Here's the drawing with two shaded views (mm, measured from the low corner). I have some questions. A direction names the side the tool comes from. Round coordinates to 2 decimals unless told otherwise and drop trailing zeros. Order: outer loops, then holes, each group sorted by start corner. A loop starts at its lowest first (then second) coordinate and runs counter-clockwise, first axis right, second up. Notation, with made-up numbers: M 71,33.25 L 108,33.25 A21 ccw 108,60.25 Z; hole C -39,22 d8. An arc over 180 degrees is marked long. One line per question, with ' | ' between items.
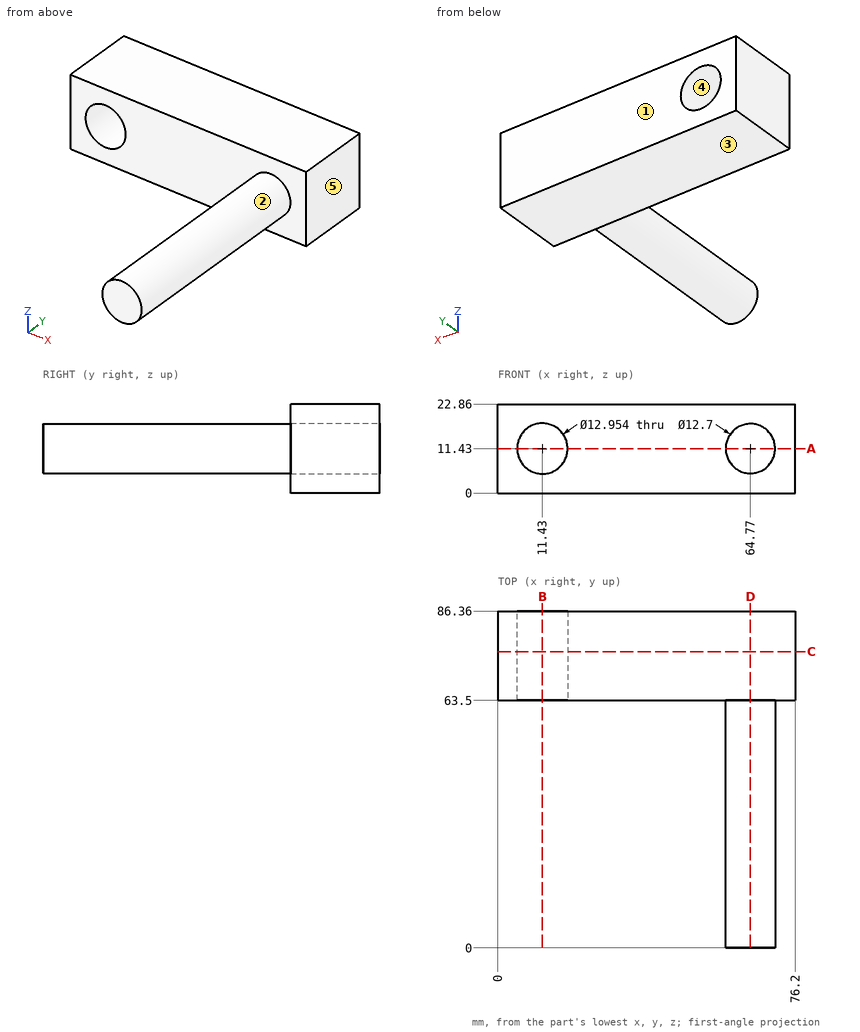
(1) Please list where these lines run through material, in increasing order: probe 1 along Z at (x, y) = (11.43, 78.25); probe 2 along X at (y, z) = (76, 10); probe 3 along Y at (x, z) = (38, 11.75). Write a range as [from, to].
Final values:
probe 1: [0, 4.95], [17.91, 22.86] | probe 2: [0, 5.11], [17.75, 76.2] | probe 3: [63.5, 86.36]
(2) Thinking about a two-plate mould opening in Z: for the marked faces 3, 4 and 5, which applies, released by +Z, released by -Z, zero draft, split by the parting line, or undercut?
Final values:
face 3: released by -Z | face 4: undercut | face 5: zero draft
(3) Will these pins go through, and if not, where does the flat tip stop? pin 1 Ø10 at (x, z) = (26, 3) entering from -Y; pin 2 Ø2 at (x, y) = (61.5, 14) entering from -Z; pin 3 Ø10 at (y, z) = (56.5, 6.5) entering from +X.
Final values:
pin 1: y = 63.5 | pin 2: z = 5.5 | pin 3: x = 71.12
(4) If we section it at A-A on z = 11.43: Please give me the cut outline in (x, y).
Final values:
outline: M 0,63.5 L 4.95,63.5 L 4.95,86.36 L 0,86.36 Z; M 17.91,63.5 L 58.42,63.5 L 58.42,0 L 71.12,0 L 71.12,63.5 L 76.2,63.5 L 76.2,86.36 L 17.91,86.36 Z
(5) If we section it at C-C on y = 76: Please give me the cut outline in (x, z), plus the area to 3 significant figures.
Final values:
outline: M 0,0 L 76.2,0 L 76.2,22.86 L 0,22.86 Z; hole C 11.43,11.43 d12.95 | area: 1,610 mm^2
(6) If we section it at B-B on x = 11.43: Please give me the cut outline in (y, z), plus the area to 3 significant figures.
Final values:
outline: M 63.5,0 L 86.36,0 L 86.36,4.95 L 63.5,4.95 Z; M 63.5,17.91 L 86.36,17.91 L 86.36,22.86 L 63.5,22.86 Z | area: 226 mm^2
(7) On a 3-axis mill with a long thin cutter (end or side, diameter ignored), from which of +Z, -Z, +X, -X, +Y, -Y can I reach the whole of each face in a straight line? I mean the marked faces 1 and 2. Say none if no direction works.
Final values:
face 1: +Z, -Z, +X, -X, +Y | face 2: -Y
(8) If we section it at D-D on x = 64.77: Please give me the cut outline in (y, z).
Final values:
outline: M 0,5.08 L 63.5,5.08 L 63.5,0 L 86.36,0 L 86.36,22.86 L 63.5,22.86 L 63.5,17.78 L 0,17.78 Z
